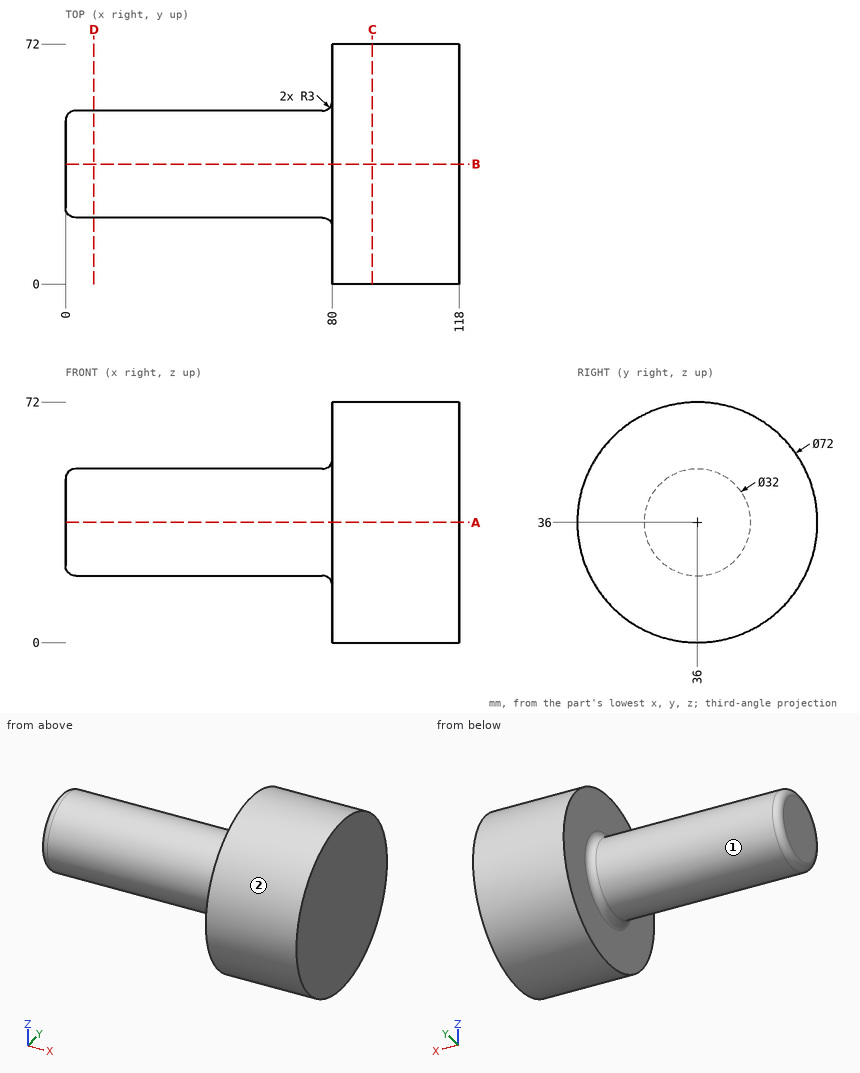
Print and shaded views of the part. All mm, measured from the part's lowest x, y and z. A direction names the side the tool comes from. Coordinates: 2 decimals unless noted, no trailing zeros. Order: outer loops, then holes, each group sorted by start corner. A loop starts at its lowest first (then second) coordinate and runs counter-clockwise, first axis right, second up. Notation, with made-up numbers: (86.5, -16.5) - (120.5, -16.5) arc R24 cw to (120.5, 9.5) - close; hole circle Ø5 at (-0.5, -32). An arc over 180 degrees is marked (long way). Put each result on its own line as item: value.
1. Saw through at A-A (z = 36). Write the cut outline in (x, y).
Answer sheet:
outline: (0, 23) arc R3 ccw to (3, 20) - (77, 20) arc R3 cw to (80, 17) - (80, 0) - (118, 0) - (118, 72) - (80, 72) - (80, 55) arc R3 cw to (77, 52) - (3, 52) arc R3 ccw to (0, 49) - close
2. Probe line 1 along X through (y, z) = (63, 19.5); line 2 along Y through (x, z) = (63, 33); line 3 along Y through (x, z) = (94, 22). List the from-to ranges inside material, lowest first. Write a range as [from, to].
Answer sheet:
line 1: x = [80, 118]
line 2: y = [20.28, 51.72]
line 3: y = [2.83, 69.17]
3. Tool access for the marked faces 1 and 2: list every direction of +Z, -Z, +X, -X, +Y, -Y with a clear straight run to the whole face (end or side of a thin tool).
Answer sheet:
face 1: -X
face 2: +X, -X
4. Saw through at D-D (x = 8.5). Write the cut outline in (y, z).
Answer sheet:
outline: circle Ø32 at (36, 36)
5. Drop flat-ended pins along their axis: P1, Ø21.5, axis at y = 21, z = 48, coming from the -X side; P2, Ø4, axis at x = 79.5, y = 45, coming from the +Z side; P3, Ø1, axis at x = 45, z = 50.5, coming from the +Y side; P4, Ø6, axis at x = 83.5, z = 36.5, coming from the +Y side. Give the stop position or say it passes through.
Answer sheet:
P1: stops at x = 0
P2: stops at z = 71.3
P3: stops at y = 43.75
P4: stops at y = 72
6. Saw through at C-C (x = 92). Write the cut outline in (y, z).
Answer sheet:
outline: circle Ø72 at (36, 36)
